from build123d import *

# Parameters (mm, degrees)
ESQUISSE1_R              = 100
BOSS_EXTRU_1_DEPTH       = 3
D_GAGEMENT_M31_OUTLINE_R = 1.7
D_GAGEMENT_M31_DEPTH     = 3
ENL_V_MAT_EXTRU_1_REACH  = 143.453
ESQUISSE5_R              = 1.25


# Read off the part's stored shape, not the designer's step: Dégagement M31
with BuildPart() as part:
    # Esquisse1 → Boss.-Extru.1 (new body)
    with BuildSketch(Plane.XY):
        Circle(ESQUISSE1_R)
    extrude(amount=BOSS_EXTRU_1_DEPTH)

    # Dégagement M31 outline → Dégagement M31 (cut)
    with BuildSketch(Plane.XY):
        with Locations((9.510565163, 3.090169944)):
            Circle(D_GAGEMENT_M31_OUTLINE_R)
        with Locations((5.877852523, -8.090169944)):
            Circle(D_GAGEMENT_M31_OUTLINE_R)
        with Locations((-5.877852523, -8.090169944)):
            Circle(D_GAGEMENT_M31_OUTLINE_R)
        with Locations((-9.510565163, 3.090169944)):
            Circle(D_GAGEMENT_M31_OUTLINE_R)
        with Locations((0, 10)):
            Circle(D_GAGEMENT_M31_OUTLINE_R)
    extrude(amount=D_GAGEMENT_M31_DEPTH, mode=Mode.SUBTRACT)

    # Esquisse5 → Enlèv. mat.-Extru.1 (cut, up to next)
    with BuildSketch(Plane.XY.offset(3), mode=Mode.PRIVATE) as enl_v_mat_extru_1_sk1:
        with Locations((17.633557569, -24.270509831)):
            Circle(ESQUISSE5_R)
    enl_v_mat_extru_1_tool1 = extrude(enl_v_mat_extru_1_sk1.sketch, amount=-ENL_V_MAT_EXTRU_1_REACH, mode=Mode.PRIVATE) & part.part
    # Esquisse5 → Enlèv. mat.-Extru.1 (cut, up to next)
    with BuildSketch(Plane.XY.offset(3), mode=Mode.PRIVATE) as enl_v_mat_extru_1_sk2:
        with Locations((-17.633557569, 24.270509831)):
            Circle(ESQUISSE5_R)
    enl_v_mat_extru_1_tool2 = extrude(enl_v_mat_extru_1_sk2.sketch, amount=-ENL_V_MAT_EXTRU_1_REACH, mode=Mode.PRIVATE) & part.part
    add(enl_v_mat_extru_1_tool1.solids().sort_by_distance((17.633558, -24.27051, 3))[0], mode=Mode.SUBTRACT)
    add(enl_v_mat_extru_1_tool2.solids().sort_by_distance((-17.633558, 24.27051, 3))[0], mode=Mode.SUBTRACT)


solid = part.part
Could you check a few things on this model? Use its own coordinates, in mm. Give positions to 0.01 mm unless a question says otherwise; leave off trailing zeros. Write each loop counter-clockwise with the first axis right and the second up, starting at its lowest first coordinate (ties: lowest second). Pieces come first, ordered by that corner, then holes. Notation, with made-up numbers: (-5.75, -13) -> (45.25, -13) arc R30 cw to (45.25, 21) -> close; hole circle Ø3 at (69, 18). An arc over 180 degrees is marked (long way). Write each question's results on one line, items separated by ' | '. Start each with the question number.
Q1. Suppose I cut it at C-C, the plane x = -72.5. List the corners of the cut face in (y, z) for me, and give its area (3 significant figures).
Q2. I'm going to push flat-ended pins straight in: pin 1 Ø1.5 at (x, z) = (-17.5, 2) entering from -Y; pin 2 Ø1.5 at (x, z) = (17.5, 1) entering from +Y. Where does each tip first touch, or does it pass through?
Q3. Suppose I cut it at A-A, the plane z = 1.3. List the corners of the cut face in (x, y) for me, and give its area (3 significant figures).
Q4. Suppose I cut it at B-B, the plane y = 74. List the corners of the cut face in (x, z) for me, and give its area (3 significant figures).
Q5. I need wall thicknesses on probe 1 along X at (y, z) = (3, 2.4); probe 2 along Y at (x, z) = (0, 1.2); probe 3 along X at (y, z) = (85, 0.3). Which ranges of each line are inside material? Lowest first, please.
Outcome:
1) outline: (-68.87, 0) -> (68.87, 0) -> (68.87, 3) -> (-68.87, 3) -> close | area: 413 mm2
2) pin 1: y = -98.59 | pin 2: y = 98.59
3) outline: circle Ø200 at (0, 0); hole circle Ø2.5 at (-17.63, 24.27); hole circle Ø3.4 at (-9.51, 3.09); hole circle Ø3.4 at (-5.88, -8.09); hole circle Ø3.4 at (0, 10); hole circle Ø3.4 at (5.88, -8.09); hole circle Ø3.4 at (9.51, 3.09); hole circle Ø2.5 at (17.63, -24.27) | area: 31,400 mm2
4) outline: (-67.26, 0) -> (67.26, 0) -> (67.26, 3) -> (-67.26, 3) -> close | area: 404 mm2
5) probe 1: -99.95 to -11.21, -7.81 to 7.81, 11.21 to 99.95 | probe 2: -100 to 8.3, 11.7 to 100 | probe 3: -52.68 to 52.68
